Can you work these out from the model? Positions are in its coordinate system, mm. A direction names the side the tool comes from. Give positions to 0.01 mm unless a question says otherwise; leave off trailing zeros. Loops run counter-clockwise (first coordinate to the right, second up) from the corner with the lowest first, then second, coordinate; pieces in that order, holes last. Notation, with made-up numbers: (-1, -33) -> (42, -33) arc R11 ccw to (42, -29) -> close; hole circle Ø3 at (76, 68). An arc over 180 degrees is marked (long way). Return JSON: item names as keys, results as strings. Group by question number.
Q1. Thinking about a two-plate mould opening in X: for faces 4 (the flat face through (-4.268, -4, 23)), 5 (the cylindrical face through (-15.05, 7.65, 47.03)), 6 (the flat face through (-17, -3, 57.15)), which applies, pulls with the +X half, pulls with the -X half, needs draft (parallel to the pull), parting line crosses it, or undercut?
Q2. Will these pins go through, and if not, where does the flat tip stop? pin 1 (6.5 mm diameter, centred on x = -12.5, z = 7, fed in from +Y); pin 2 (10 mm diameter, centred on x = -25.5, y = -9, fed in from +Z); pin 3 (8.5 mm diameter, centred on x = -16.86, z = 41.28, fed in from -Y); pin 4 (4.5 mm diameter, centred on x = -18.5, y = -4, fed in from -Z).
Q3. Which directions (+Z, -Z, +X, -X, +Y, -Y) give clear straight access to the entire face, cutting with the end or side of a thin tool? Please do faces 1 (the flat face through (-15, 6.038, 46)), 2 (the flat face through (-17, 6.038, 11)), 3 (the cylindrical face through (-13.17, -6.31, 14.88)).
Q4. I need wall thicknesses on line 1 along Y through (x, z) = (-17.25, 24); line 2 along X through (y, z) = (-3.5, 23.5); line 3 along Y through (x, z) = (-17.75, 47). Which ranges of each line are inside material? Lowest first, please. Write a range as [from, to].
Q5. Suppose I cut it at C-C, the plane z = 12. Please give me the cut outline in (x, y).
Q6. Suppose I cut it at D-D, the plane x = -11.5. Please give me the cut outline in (y, z) (3 decimals).
Q7. Suppose I cut it at A-A, the plane z = 39.5. Please give me the cut outline in (x, y), and give its area (3 significant figures).
```python
from build123d import *

# Parameters (mm, degrees)
SKETCH1_W           = 25.191803279
SKETCH1_H           = 25.4
BOSS_EXTRUDE1_DEPTH = 57.15
SKETCH2_R           = 4.696654448
CUT_EXTRUDE1_DEPTH  = 30.1752
SKETCH3_W           = 22.225
SKETCH3_H           = 3.175
CUT_EXTRUDE2_DEPTH  = 30.1752
SKETCH11_R          = 6.0325
CUT_EXTRUDE5_DEPTH  = 3.175
SKETCH12_R          = 4.7625
CUT_EXTRUDE6_DEPTH  = 69.029075152
FILLET1_R           = 10.16
FILLET2_R           = 10.16


with BuildPart() as part:
    # Sketch1 → Boss-Extrude1 (new body)
    with BuildSketch(Plane.XY):
        with Locations((-16.863934427, -3.487295082)):
            Rectangle(SKETCH1_W, SKETCH1_H)
    extrude(amount=BOSS_EXTRUDE1_DEPTH)

    # Sketch2 → Cut-Extrude1 (cut)
    with BuildSketch(Plane(origin=(0, 0, 0), x_dir=(-1, 0, 0), z_dir=(0, 0, -1))):
        with Locations((16.89886731, -3.452362198)):
            Circle(SKETCH2_R)
    extrude(amount=-CUT_EXTRUDE1_DEPTH, mode=Mode.SUBTRACT)

    # Sketch3 → Cut-Extrude2 (cut)
    with BuildSketch(Plane(origin=(-4.268032787, 0, 0), x_dir=(0, 0, -1), z_dir=(1, 0, 0))):
        with Locations((-11.1125, 7.625204918)):
            Rectangle(SKETCH3_W, SKETCH3_H)
    extrude(amount=-CUT_EXTRUDE2_DEPTH, mode=Mode.SUBTRACT)

    # Sketch11 → Cut-Extrude5 (cut)
    with BuildSketch(Plane(origin=(0, 9.212704918, 0), x_dir=(1, 0, 0), z_dir=(0, 1, 0))):
        with Locations(Location((-16.863934426, -41.275, 0), (0, 0, 270))):
            Circle(SKETCH11_R)
    extrude(amount=-CUT_EXTRUDE5_DEPTH, mode=Mode.SUBTRACT)

    # Sketch12 → Cut-Extrude6 (cut, through all)
    with BuildSketch(Plane(origin=(0, 6.037704918, 0), x_dir=(1, 0, 0), z_dir=(0, 1, 0))):
        with Locations(Location((-16.863934426, -41.275, 0), (0, 0, 270))):
            Circle(SKETCH12_R)
    extrude(amount=-CUT_EXTRUDE6_DEPTH, mode=Mode.SUBTRACT)

    # Fillet1
    fillet1_edges = [part.edges().sort_by_distance(p)[0] for p in [
        (-4.268032787, -3.487295082, 57.15),
    ]]
    fillet(fillet1_edges, radius=FILLET1_R)

    # Fillet2
    fillet2_edges = [part.edges().sort_by_distance(p)[0] for p in [
        (-29.459836066, -3.487295082, 57.15),
    ]]
    fillet(fillet2_edges, radius=FILLET2_R)


solid = part.part
```
Ans:
{
 "1": {"face 4": "pulls with the +X half", "face 5": "undercut", "face 6": "needs draft"},
 "2": {"pin 1": "stops at y = 6.04", "pin 2": "stops at z = 57.08", "pin 3": "passes through", "pin 4": "stops at z = 30.18"},
 "3": {"face 1": "+Y", "face 2": "-Z, +X, -X, +Y", "face 3": "-Z"},
 "4": {"line 1": "y = [-16.19, -8.14], [1.23, 9.21]", "line 2": "x = [-29.46, -21.6], [-12.2, -4.27]", "line 3": "y = [-16.19, 6.04]"},
 "5": {"outline": "(-29.46, -16.19) -> (-4.27, -16.19) -> (-4.27, 6.04) -> (-29.46, 6.04) -> close; hole circle Ø9.39 at (-16.9, -3.45)"},
 "6": {"outline": "(-16.187, 0) -> (6.038, 0) -> (6.038, 22.225) -> (9.213, 22.225) -> (9.213, 38.515) -> (6.038, 38.515) -> (6.038, 44.035) -> (9.213, 44.035) -> (9.213, 56.719) -> (-16.187, 56.719) -> close"},
 "7": {"outline": "(-29.46, -16.19) -> (-21.28, -16.19) -> (-21.28, 6.04) -> (-22.63, 6.04) -> (-22.63, 9.21) -> (-29.46, 9.21) -> close; (-12.44, -16.19) -> (-4.27, -16.19) -> (-4.27, 9.21) -> (-11.1, 9.21) -> (-11.1, 6.04) -> (-12.44, 6.04) -> close", "area": "407 mm^2"}
}
